from build123d import *

# Parameters (mm, degrees)
BOSS_EXTRUDE1_DEPTH = 914.4
CUT_EXTRUDE1_REACH  = 103.6
SKETCH2_R           = 11.1125


with BuildPart() as part:
    # Sketch1 → Boss-Extrude1 (new body, symmetric)
    with BuildSketch(Plane.XY):
        with BuildLine():
            Line((0, 0), (0, 152.4))
            Line((0, 152.4), (0.00508, 152.4))
            ThreePointArc((0.00508, 152.4), (8.981744019, 148.681744019), (12.7, 139.70508))
            Line((12.7, 139.70508), (12.7, 25.4))
            ThreePointArc((12.7, 25.4), (16.419743879, 16.419743879), (25.4, 12.7))
            Line((25.4, 12.7), (88.90508, 12.7))
            ThreePointArc((88.90508, 12.7), (97.881744019, 8.981744019), (101.6, 0.00508))
            Line((101.6, 0.00508), (101.6, 0))
            Line((101.6, 0), (0, 0))
        make_face()
    extrude(amount=BOSS_EXTRUDE1_DEPTH, both=True)

    # Sketch2 → Cut-Extrude1 (cut, up to next)
    with BuildSketch(Plane.ZY, mode=Mode.PRIVATE) as cut_extrude1_sk1:
        with Locations((346.964, 50.8)):
            Circle(SKETCH2_R)
    cut_extrude1_tool1 = extrude(cut_extrude1_sk1.sketch, amount=-CUT_EXTRUDE1_REACH, mode=Mode.PRIVATE) & part.part
    add(cut_extrude1_tool1.solids().sort_by_distance((0, 50.8, 346.964))[0], mode=Mode.SUBTRACT)
    # Sketch2 → Cut-Extrude1 (cut, up to next)
    with BuildSketch(Plane.ZY, mode=Mode.PRIVATE) as cut_extrude1_sk2:
        with Locations((-347.218, 50.8)):
            Circle(SKETCH2_R)
    cut_extrude1_tool2 = extrude(cut_extrude1_sk2.sketch, amount=-CUT_EXTRUDE1_REACH, mode=Mode.PRIVATE) & part.part
    add(cut_extrude1_tool2.solids().sort_by_distance((0, 50.8, -347.218))[0], mode=Mode.SUBTRACT)
    # Sketch2 → Cut-Extrude1 (cut, up to next)
    with BuildSketch(Plane.ZY, mode=Mode.PRIVATE) as cut_extrude1_sk3:
        with Locations((346.964, 101.791886097)):
            Circle(SKETCH2_R)
    cut_extrude1_tool3 = extrude(cut_extrude1_sk3.sketch, amount=-CUT_EXTRUDE1_REACH, mode=Mode.PRIVATE) & part.part
    add(cut_extrude1_tool3.solids().sort_by_distance((0, 101.791886, 346.964))[0], mode=Mode.SUBTRACT)
    # Sketch2 → Cut-Extrude1 (cut, up to next)
    with BuildSketch(Plane.ZY, mode=Mode.PRIVATE) as cut_extrude1_sk4:
        with Locations((-347.218, 101.6)):
            Circle(SKETCH2_R)
    cut_extrude1_tool4 = extrude(cut_extrude1_sk4.sketch, amount=-CUT_EXTRUDE1_REACH, mode=Mode.PRIVATE) & part.part
    add(cut_extrude1_tool4.solids().sort_by_distance((0, 101.6, -347.218))[0], mode=Mode.SUBTRACT)


solid = part.part
Work out the finished part from the listing and answer in its coordinate system (mm). A direction names the side the tool comes from. Give positions to 0.01 mm unless a question says otherwise; leave off trailing zeros. Loops run counter-clockwise (first coordinate to the right, second up) from the corner with the lowest first, then second, coordinate; pieces in that order, holes last. Notation, with made-up numbers: (63, 4) -> (91, 4) arc R31 cw to (91, 36) -> close; hole circle Ø8 at (22, 36.25). An arc over 180 degrees is marked (long way). Use a Markdown table: item, result. Add a question column.
1. Section B-B on x = 52 is taken. Determine the outline of the cut face in (y, z).
2. Find the intervals of material crossed by probe 1 along Y at (x, z) = (74, 449.5); probe 2 along X at (y, z) = (10, -168), in increasing order.
3. Flat-ended cylindrical pins translate along their axes: pin 1 Ø10 at (x, z) = (33.5, 459) entering from +Y; pin 2 Ø3 at (y, z) = (44.5, -525) entering from +X. Find the tip coordinate at first contact, or state that the pin passes through.
4. For faces 1 (the flat face through (57, 12.7, 13)), 2 (the flat face through (10, 54, 914.4)), determine the directions among +Z, -Z, +X, -X, +Y, -Y from which every point of the face is accessible in a straight line to the end or side of a thin tool.
Results below:
| question | item | result |
|---|---|---|
| 1 | outline | (0, -914.4) -> (12.7, -914.4) -> (12.7, 914.4) -> (0, 914.4) -> close |
| 2 | probe 1 | y = 0 to 12.7 |
| 2 | probe 2 | x = 0 to 96.73 |
| 3 | pin 1 | stops at y = 12.7 |
| 3 | pin 2 | stops at x = 12.7 |
| 4 | face 1 | +Z, -Z, +X, +Y |
| 4 | face 2 | +Z, +X, -X, +Y, -Y |
